```python
from build123d import *

# Parameters (mm, degrees)
F0_R     = 25.4
F1_DEPTH = 6.35
F2_R     = 22.225
F3_DEPTH = 12.7
F4_R     = 6.35
F5_DEPTH = 19.051
F6_R     = 25.4
F7_DEPTH = 6.35


with BuildPart() as f1:
    # F0 (on Front) → F1 (new body)
    with BuildSketch(Plane.XZ):
        Circle(F0_R)
    extrude(amount=F1_DEPTH)

    # F2 (on face) → F3 (join)
    with BuildSketch(Plane.XZ.offset(6.35)):
        Circle(F2_R)
    extrude(amount=F3_DEPTH)

    # F4 (on face) → F5 (cut, through all)
    with BuildSketch(Plane.XZ.offset(19.05)):
        Circle(F4_R)
    extrude(amount=-F5_DEPTH, mode=Mode.SUBTRACT)

    # F6 (on face) → F7 (join)
    with BuildSketch(Plane.XZ.offset(19.05)):
        Circle(F6_R)
    extrude(amount=F7_DEPTH)


solid = f1.part
```
Input: part model. Units: mm. Frame: model coordinates. A direction names the side the tool comes from. Give positions to 0.01 mm unless a question says otherwise; leave off trailing zeros. Loops run counter-clockwise (first coordinate to the right, second up) from the corner with the lowest first, then second, coordinate; pieces in that order, holes last.
1) Reachability of faces 1 (the cylindrical face through (-5.506, -22.181, -24.796)), 2 (the cylindrical face through (21.199, -12.611, 6.676)) from +Z, -Z, +X, -X, +Y, -Y: full face, straight path, thin tool, end or side. Return the list, or none.
A:
face 1: +Y, -Y
face 2: none
2) Section query D-D on y = -24. Return the cut outline in (x, z).
A:
outline: circle Ø50.8 at (0, 0)
3) Mould query, pull axis Z, two halves, no side actions, for faces 3 (the flat face through (5, 0, -5)), 4 (the cylindrical face through (-5.506, -3.131, -24.796)), 5 (the flat face through (0, -19.05, 0)), 6 (the cylindrical face through (-1.38, -9.66, -6.2)). Classes: released by +Z, released by -Z, zero draft, split by the parting line, or undercut.
A:
face 3: zero draft
face 4: split by the parting line
face 5: undercut
face 6: undercut
4) Contact query for flat-ended pins moving along their axis: pin 1 (3 mm diameter, centred on x = -2, y = -9, fed in from +Z); pin 2 (6.5 mm diameter, centred on x = -1.5, z = -0.5, fed in from +Y); pin 3 (3 mm diameter, centred on y = -13, z = -13, fed in from +X). Output: stop coordinate, or through.
A:
pin 1: stops at z = 22.22
pin 2: stops at y = -19.05
pin 3: stops at x = 19.02
5) Section query C-C on y = -14. Return the cut outline in (x, z) (3 decimals), and give its area (3 significant figures).
A:
outline: circle Ø44.45 at (0, 0); hole circle Ø12.7 at (0, 0)
area: 1,430 mm2
6) Section query B-B on z = 0. Return the cut outline in (x, y) (3 decimals), and give its area (3 significant figures).
A:
outline: (-25.4, -25.4) - (25.4, -25.4) - (25.4, -19.05) - (22.225, -19.05) - (22.225, -6.35) - (25.4, -6.35) - (25.4, 0) - (6.35, 0) - (6.35, -19.05) - (-6.35, -19.05) - (-6.35, 0) - (-25.4, 0) - (-25.4, -6.35) - (-22.225, -6.35) - (-22.225, -19.05) - (-25.4, -19.05) - close
area: 968 mm2
7) Line query: L1, parallel to Z at x = 0, y = -6.25; L2, parallel to Y at x = -20.5, z = 12; L3, parallel to Z at x = 0, y = -12.75 (3 decimals). Output: solid intervals per line, ascending.
A:
L1: z = -25.4 to -6.35, 6.35 to 25.4
L2: y = -25.4 to -19.05, -6.35 to 0
L3: z = -22.225 to -6.35, 6.35 to 22.225
8) Section query A-A on x = 0. Return the cut outline in (y, z) (3 decimals), and give its area (3 significant figures).
A:
outline: (-25.4, -25.4) - (-19.05, -25.4) - (-19.05, -22.225) - (-6.35, -22.225) - (-6.35, -25.4) - (0, -25.4) - (0, -6.35) - (-19.05, -6.35) - (-19.05, 6.35) - (0, 6.35) - (0, 25.4) - (-6.35, 25.4) - (-6.35, 22.225) - (-19.05, 22.225) - (-19.05, 25.4) - (-25.4, 25.4) - close
area: 968 mm2
